Part model, mm, in its own coordinate system. Round coordinates to 2 decimals unless told otherwise and drop trailing zeros. Loops run counter-clockwise (first coordinate to the right, second up) from the corner with the lowest first, then second, coordinate; pieces in that order, holes last. Notation, with made-up numbers: M -32,2 L 12,2 A25 ccw 12,26 Z; hole C 86,82 d6. An arc over 180 degrees is marked long. Put each result on its own line as item: value. Start each with the question number.
1) Drop flat-ended pins along their axis: pin 1 Ø3 at (x, y) = (44.5, -63.5) entering from +Z; pin 2 Ø4 at (x, y) = (172.4, -49.89) entering from +Z. Give the stop position or say it passes through.
2) Slice it at B-B on x = 146.5. Give the cut face in (y, z), then the cut area to 3 significant figures.
3) Slice it at A-A on z = 0.3. State how many separate pieces and enclosed holes the cut face has, then the cut area to 3 significant figures.
4) Probe line 1 along Y through (x, z) = (5.6, 0.45); line 2 along X through (y, z) = (-70.5, 0.3); line 3 along X through (y, z) = (-60, 0.7). List the from-to ranges inside material, lowest first.
Autodesk Inventor part; units mm, degrees
ref_plane "YZ Plane" through (0, 0, 0) normal (1, 0, 0) x (0, 1, 0)
ref_plane "XZ Plane" through (0, 0, 0) normal (0, 1, 0) x (-1, 0, 0)
ref_plane "XY Plane" through (0, 0, 0) normal (0, 0, 1) x (1, 0, 0)
ref_plane "Work Plane1" through (0, 0, 0) normal (0, 0, 1) x (1, 0, 0)
sketch "Sketch1" plane through (0, 0, 0) normal (0, 0, 1) x (1, 0, 0)
  circle A0 centre (118.7, -21.5445) radius 2.5
  circle A1 centre (113.95, -8.8843) radius 2.5
  circle A2 centre (64.05, -19.8657) radius 2.5
  circle A3 centre (59.3, -7.2055) radius 2.5
  circle A4 centre (64.05, -8.8843) radius 2.5
  circle A5 centre (59.3, -21.5445) radius 2.5
  circle A6 centre (118.7, -7.2055) radius 2.5
  circle A7 centre (113.95, -19.8657) radius 2.5
  line L0 (84.5, 12.4325) -> (84.5, -11.5675)
  line L1 (84.5, -11.5675) -> (72.5, -11.5675)
  line L2 (72.5, -11.5675) -> (72.5, 4.5875)
  circle A8 centre (69.5, 4.5875) radius 3
  line L3 (72.5, 4.5875) -> (72.5, 12.4325)
  line L4 (72.5, 12.4325) -> (84.5, 12.4325)
  arc A9 (105.5, 4.2836) -> (105.5, 4.8914) centre (108.4846, 4.5875) ccw
  line L5 (105.5, 4.2836) -> (105.5, -11.5675)
  line L6 (105.5, -11.5675) -> (93.5, -11.5675)
  line L7 (93.5, -11.5675) -> (93.5, 12.4325)
  line L8 (93.5, 12.4325) -> (105.5, 12.4325)
  line L9 (105.5, 12.4325) -> (105.5, 4.8914)
  circle A10 centre (108.4462, 27.5) radius 3
  circle A11 centre (69.5, 27.5) radius 3
  circle A12 centre (89, 0.9661) radius 3
  circle A13 centre (89, 29.5) radius 3
  arc A14 (175, 0) -> (178, -3) centre (175, -3) ccw
  line L10 (175, 0) -> (112.5, 0)
  line L11 (112.5, 0) -> (112.5, 55)
  line L12 (112.5, 55) -> (65.5, 55)
  line L13 (65.5, 55) -> (65.5, 0)
  line L14 (65.5, 0) -> (3, 0)
  arc A15 (0, -3) -> (3, 0) centre (3, -3) ccw
  line L15 (0, -3) -> (0, -25.75)
  arc A16 (3, -28.75) -> (0, -25.75) centre (3, -25.75) ccw
  line L16 (3, -28.75) -> (175, -28.75)
  arc A17 (178, -25.75) -> (175, -28.75) centre (175, -25.75) ccw
  line L17 (178, -25.75) -> (178, -3)
  circle A18 centre (3, -25.75) radius 2.3
  circle A19 centre (3, -3) radius 2.3
  circle A20 centre (3, -74.8889) radius 2.3
  line L18 (0, 0) -> (6, 0)
  line L19 (0, -77.8889) -> (0, 0)
  line L20 (0, -77.8889) -> (6, -77.8889)
  line L21 (6, -71.8889) -> (6, -77.8889)
  line L22 (6, -71.8889) -> (1.6, -71.8889)
  line L23 (1.6, -71.8889) -> (1.6, -56.7889)
  line L24 (1.6, -56.7889) -> (9.6, -56.7889)
  line L25 (9.6, -44.7889) -> (9.6, -56.7889)
  line L26 (3, -44.7889) -> (9.6, -44.7889)
  line L27 (3, -28.75) -> (3, -44.7889)
  line L28 (3, -28.75) -> (6, -28.75)
  line L29 (6, -28.75) -> (6, -22.75)
  line L30 (6, -22.75) -> (3, -22.75)
  line L31 (3, -6) -> (3, -22.75)
  line L32 (3, -6) -> (6, -6)
  line L33 (6, -6) -> (6, 0)
  circle A21 centre (5.6, -52.7889) radius 2.6
  circle A22 centre (175, -3) radius 2.3
  circle A23 centre (175, -25.75) radius 2.3
  line L34 (175, -28.75) -> (175, -41.8889)
  line L35 (168.4, -41.8889) -> (175, -41.8889)
  line L36 (168.4, -53.8889) -> (168.4, -41.8889)
  line L37 (175, -53.8889) -> (168.4, -53.8889)
  line L38 (175, -53.8889) -> (175, -71.8889)
  line L39 (175, -71.8889) -> (172, -71.8889)
  line L40 (172, -71.8889) -> (172, -77.8889)
  line L41 (178, -77.8889) -> (172, -77.8889)
  line L42 (178, -77.8889) -> (178, 0)
  line L43 (178, 0) -> (172, 0)
  line L44 (172, 0) -> (172, -6)
  line L45 (172, -6) -> (175, -6)
  line L46 (175, -6) -> (175, -22.75)
  line L47 (175, -22.75) -> (172, -22.75)
  line L48 (172, -22.75) -> (172, -28.75)
  line L49 (172, -28.75) -> (175, -28.75)
  circle A24 centre (175, -74.8889) radius 2.3
  circle A25 centre (172.4, -49.8889) radius 2.6
  line L50 (156.2, -70.4889) -> (156.2, -59.9889)
  line L51 (166.7, -59.9889) -> (156.2, -59.9889)
  line L52 (166.7, -59.9889) -> (166.7, -70.4889)
  line L53 (156.2, -70.4889) -> (166.7, -70.4889)
  line L54 (149, -59.8889) -> (149, -70.8889)
  line L55 (149, -70.8889) -> (136.35, -70.8889)
  line L56 (136.35, -70.8889) -> (136.35, -59.8889)
  line L57 (136.35, -59.8889) -> (149, -59.8889)
  line L58 (135, -53.8889) -> (135, -71.8889)
  line L59 (135, -71.8889) -> (175, -71.8889)
  line L60 (175, -71.8889) -> (175, -53.8889)
  line L61 (175, -53.8889) -> (135, -53.8889)
  circle A26 centre (137.85, -56.7389) radius 1.5
  circle A27 centre (172.15, -56.7389) radius 1.5
  line L62 (31.25, -62.8889) -> (31.25, -73.8889)
  line L63 (31.25, -73.8889) -> (57.25, -73.8889)
  line L64 (57.25, -73.8889) -> (57.25, -62.8889)
  line L65 (57.25, -62.8889) -> (31.25, -62.8889)
  line L66 (9.6, -56.7889) -> (23.3, -56.7889)
  line L67 (23.3, -56.7889) -> (23.3, -59.8889)
  line L68 (23.3, -59.8889) -> (23.3, -65.1889)
  line L69 (3, -71.8889) -> (23.3, -71.8889)
  line L70 (23.3, -61.8889) -> (23.3, -74.8889)
  line L71 (30.25, -61.8889) -> (30.25, -74.8889)
  line L72 (30.25, -74.8889) -> (58.25, -74.8889)
  line L73 (58.25, -74.8889) -> (58.25, -61.8889)
  line L74 (58.25, -61.8889) -> (30.25, -61.8889)
  line L75 (150, -58.8889) -> (150, -71.8889)
  line L76 (150, -71.8889) -> (135.35, -71.8889)
  line L77 (135.35, -71.8889) -> (135.35, -58.8889)
  line L78 (135.35, -58.8889) -> (150, -58.8889)
  line L79 (155.2, -58.9889) -> (155.2, -71.4889)
  line L80 (155.2, -71.4889) -> (167.7, -71.4889)
  line L81 (167.7, -71.4889) -> (167.7, -58.9889)
  line L82 (167.7, -58.9889) -> (155.2, -58.9889)
  line L83 (0, -28.75) -> (178, -28.75)
  line L84 (178, -28.75) -> (178, -77.8889)
  line L85 (178, -77.8889) -> (0, -77.8889)
  line L86 (0, -77.8889) -> (0, -28.75)
  point P0 (3, -28.75)
  point P1 (175, -28.75)
  point P2 (135.35, -71.8889)
  dimension "d0" = 1
  dimension "d1" = 1
  dimension "d2" = 1
extrude "Extrusion1" add sketch "Sketch1" along normal blind 2 contours L42 L41 L40 L39 L38 L37 L36 L35 L34 L83 | L34 L35 L36 L61 L58 L59 L40 L85 L21 L69 L70 L68 L67 L66 L25 L26 L27 L16 | L27 L26 L25 L24 L23 L22 L21 L20 L19 L83 | L59 L75 L78 L77 L58 L61 L37 L38 L39 | A20 | A21 | A24 | A25 | A26 | A27
sketch "Sketch2" plane through (0, 0, 2) normal (0, 0, 1) x (1, 0, 0)
  circle A0 centre (3, -25.75) radius 2.3
  circle A1 centre (3, -3) radius 2.3
  circle A2 centre (3, -74.8889) radius 2.3
  line L0 (0, 0) -> (6, 0)
  line L1 (0, -77.8889) -> (0, 0)
  line L2 (0, -77.8889) -> (6, -77.8889)
  line L3 (6, -71.8889) -> (6, -77.8889)
  line L4 (6, -71.8889) -> (1.6, -71.8889)
  line L5 (1.6, -71.8889) -> (1.6, -56.7889)
  line L6 (1.6, -56.7889) -> (9.6, -56.7889)
  line L7 (9.6, -44.7889) -> (9.6, -56.7889)
  line L8 (3, -44.7889) -> (9.6, -44.7889)
  line L9 (3, -28.75) -> (3, -44.7889)
  line L10 (3, -28.75) -> (6, -28.75)
  line L11 (6, -28.75) -> (6, -22.75)
  line L12 (6, -22.75) -> (3, -22.75)
  line L13 (3, -6) -> (3, -22.75)
  line L14 (3, -6) -> (6, -6)
  line L15 (6, -6) -> (6, 0)
  circle A3 centre (5.6, -52.7889) radius 2.6
  circle A4 centre (172.4, -49.8889) radius 2.6
  circle A5 centre (175, -3) radius 2.3
  circle A6 centre (175, -25.75) radius 2.3
  line L16 (175, -28.75) -> (175, -41.8889)
  line L17 (168.4, -41.8889) -> (175, -41.8889)
  line L18 (168.4, -53.8889) -> (168.4, -41.8889)
  line L19 (175, -53.8889) -> (168.4, -53.8889)
  line L20 (175, -53.8889) -> (175, -71.8889)
  line L21 (175, -71.8889) -> (172, -71.8889)
  line L22 (172, -71.8889) -> (172, -77.8889)
  line L23 (178, -77.8889) -> (172, -77.8889)
  line L24 (178, -77.8889) -> (178, 0)
  line L25 (178, 0) -> (172, 0)
  line L26 (172, 0) -> (172, -6)
  line L27 (172, -6) -> (175, -6)
  line L28 (175, -6) -> (175, -22.75)
  line L29 (175, -22.75) -> (172, -22.75)
  line L30 (172, -22.75) -> (172, -28.75)
  line L31 (172, -28.75) -> (175, -28.75)
  circle A7 centre (175, -74.8889) radius 2.3
  circle A8 centre (172.4, -49.8889) radius 2.6
hole "Hole1" at (5.6, -52.7889, 2) at (3, -74.8889, 2) at (175, -74.8889, 2) at (172.4, -49.8889, 2) direction (0, 0, -1) diameter 3.6 end through all countersink diameter 6 countersink angle 90
properties part number "ceil_front"
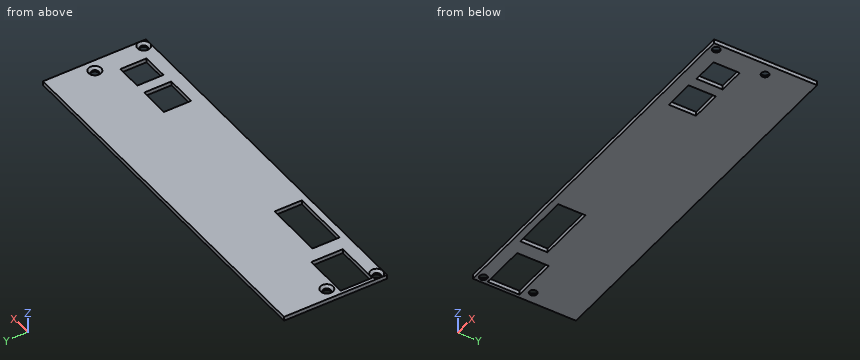
Recorded:
1. pin 1: passes through
1. pin 2: stops at z = 1
2. outline: M -77.89,0 L -71.89,0 L -71.89,2 L -77.89,2 Z; M -58.89,0 L -28.75,0 L -28.75,2 L -58.89,2 Z
2. area: 72.3 mm2
3. separate pieces: 1
3. enclosed holes: 8
3. area: 7,670 mm2
4. line 1: y = -77.89 to -71.89, -56.79 to -54.59, -50.99 to -28.75
4. line 2: x = 0 to 1.6, 23.3 to 30.25, 58.25 to 135.35, 150 to 155.2, 167.7 to 178
4. line 3: x = 0 to 1.6, 23.3 to 135.35, 150 to 155.2, 167.7 to 178
